Autodesk Inventor part; units mm, degrees
ref_plane "YZ Plane" through (0, 0, 0) normal (1, 0, 0) x (0, 1, 0)
ref_plane "XZ Plane" through (0, 0, 0) normal (0, 1, 0) x (-1, 0, 0)
ref_plane "XY Plane" through (0, 0, 0) normal (0, 0, 1) x (1, 0, 0)
sketch "Sketch1" plane through (0, 0, 0) normal (0, 0, 1) x (1, 0, 0)
  line L0 (-28.59, -15) -> (28.59, -15)
  line L1 (28.59, -15) -> (28.59, 15)
  line L2 (28.59, 15) -> (-28.59, 15)
  line L3 (-28.59, 15) -> (-28.59, -15)
  line L4 (-28.59, -15) -> (28.59, 15) construction
  line L5 (28.59, -15) -> (-28.59, 15) construction
  point P0 (0, 0)
  dimension "d0" = 57.18
  dimension "d1" = 30
extrude "Plate1" add sketch "Sketch1" along normal blind 1.5
sketch "Sketch2" plane through (-27.09, -15, 0) normal (-1, 0, 0) x (0, -1, 0)
  line L0 (-30, 0) -> (0, 0)
  line L1 (0, 0) -> (0, 40)
  line L2 (0, 40) -> (-30, 40)
  line L3 (-30, 40) -> (-30, 0)
edge flange "Flange1" height 40 angle 90 thickness 1.5 bend radius 0.31 thickness toward (-1, 0, 0) relief tear relief width 1.5 relief depth 0.75 corner gap 0.31 corner form 0 edges at (-28.59, 0, 1.5) (28.59, 0, 1.5) wall of the first edge with corners at (-27.09, 15, 0) (-27.09, -15, 0) (-27.09, -15, 40) (-27.09, 15, 40)
bend "Bend1"
corner "Corner1"
sketch "Sketch3" plane through (28.59, -15, 40) normal (1, 0, 0) x (0, 0, -1)
  circle A0 centre (15, 15) radius 9.96
  line L0 (0, 30) -> (38.19, 30)
  line L1 (38.19, 0) -> (0, 0)
  line L2 (38.19, 30) -> (12.9705, 24.751)
  line L3 (38.19, 0) -> (12.9705, 5.249)
  line L4 (0, 30) -> (0, 0)
  point P0 (40, 15)
  dimension "d13" = 19.92
  dimension "d14" = 0
  dimension "d15" = 25
sketch "Sketch19" plane through (0, 0, 1.5) normal (0, 0, 1) x (1, 0, 0)
  point P0 (0, 0)
sketch "Sketch21" plane through (-28.59, -15, 1.81) normal (-1, 0, 0) x (0, 0, 1)
  point P0 (-1.81, 15)
sketch "Sketch23" plane through (-28.59, -15, 1.81) normal (-1, 0, 0) x (0, 0, 1)
  point P0 (-1.81, 15)
sketch "Sketch25" plane through (0, 0, 1.5) normal (0, 0, 1) x (1, 0, 0)
  circle A0 centre (7.525, 7.5) radius 0.7835
  circle A1 centre (7.525, -12.5) radius 0.7835
  circle A2 centre (-7.525, -12.5) radius 0.7835
  circle A3 centre (-7.525, 7.5) radius 0.7835
  point P0 (0, 0)
hole "Hole12" at (7.525, 7.5, 1.5) at (7.525, -12.5, 1.5) at (-7.525, 7.5, 1.5) at (-7.525, -12.5, 1.5) direction (0, 0, -1) diameter 2.1 depth 1.5
extrude "Cut7" cut sketch "Sketch3" against normal blind 1.5 contours A0 L3 L1 L4 L0 L2
mirror "Mirror1" about plane through (0, 0, 0) normal (1, 0, 0) of "Cut7"
sketch "Sketch26" plane through (-28.59, -15, 1.81) normal (-1, 0, 0) x (0, 0, 1)
  circle A0 centre (30.19, 15) radius 0.7835
  circle A1 centre (23.19, 22) radius 0.7835
  circle A2 centre (23.19, 8) radius 0.7835
  circle A3 centre (16.19, 15) radius 0.7835
  point P0 (-1.81, 15)
hole "Hole13" at (-28.59, 0, 32) at (-28.59, 7, 25) at (-28.59, -7, 25) at (-28.59, 0, 18) direction (1, 0, 0) diameter 2.1 depth 1.5
sketch "Sketch27" plane through (-28.59, -15, 1.81) normal (-1, 0, 0) x (0, 0, 1)
  circle A0 centre (23.19, 15) radius 3
  point P0 (-1.81, 15)
hole "Hole14" at (-28.59, 0, 25) direction (1, 0, 0) diameter 7.2 depth 1.5
sketch "Sketch28" plane through (28.59, -15, 1.81) normal (1, 0, 0) x (0, 0, -1)
  circle A0 centre (-30.19, 15) radius 0.7835
  circle A1 centre (-23.19, 8) radius 0.7835
  circle A2 centre (-23.19, 22) radius 0.7835
  circle A3 centre (-16.19, 15) radius 0.7835
  point P0 (1.81, 15)
hole "Hole15" at (28.59, 0, 32) at (28.59, -7, 25) at (28.59, 0, 18) at (28.59, 7, 25) direction (-1, 0, 0) diameter 2.1 depth 1.5
sketch "Sketch29" plane through (28.59, -15, 1.81) normal (1, 0, 0) x (0, 0, -1)
  circle A0 centre (-23.19, 15) radius 1.75
  point P0 (1.81, 15)
hole "Hole16" at (28.59, 0, 25) direction (-1, 0, 0) diameter 5.2 depth 1.5
equation "\"d125\" = Thickness"
equation "\"d127\" = Thickness"
equation "\"d134\" = Thickness"
equation "\"d141\" = Thickness"
equation "\"d148\" = Thickness"
equation "\"d155\" = Thickness"
equation "\"d2\" = Thickness"
equation "\"d3\" = BendReliefWidth"
equation "\"d4\" = BendReliefDepth"
equation "\"d5\" = MinimumRemnant"
equation "\"d6\" = TransitionRadius"
equation "\"d9\" = BendRadius"
equation "\"d10\" = CornerReliefSize"
equation "\"d11\" = GapSize"
equation "\"d12\" = JacobiRadiusSize"
equation "\"BendReliefWidth\" = Thickness"
equation "\"BendReliefDepth\" = 0.5 * Thickness"
equation "\"CornerReliefSize\" = 4 * Thickness"
equation "\"MinimumRemnant\" = 2 * Thickness"
equation "\"TransitionRadius\" = BendRadius"
equation "\"JacobiRadiusSize\" = BendRadius"
equation "\"GapSize\" = Thickness"
properties part number "axis_14_bottom_frame" material "Aluminum 6061-AHC"
Source: CAD feature listing. Evaluate the final solid. Frame: model axes, mm. A direction names the side the tool comes from. Round coordinates to 2 decimals unless told otherwise and drop trailing zeros. Order: outer loops, then holes, each group sorted by start corner. A loop starts at its lowest first (then second) coordinate and runs counter-clockwise, first axis right, second up. Notation, with made-up numbers: (-15, 73.25) - (3, 73.25) arc R24 cw to (3, 83.25) - close; hole circle Ø8 at (47.25, 57). An arc over 180 degrees is marked (long way). Use a Markdown table: item, result. Add a question column.
1. Set-up query: faces 5 (the cylindrical face through (27.83, 6.68, 24)), 6 (the cylindrical face through (-27.83, -0.158, 21.403)), 7 (the flat face through (-27.09, 0, 14)). Return all of +Z, -Z, +X, -X, +Y, -Y with unobstructed straight access to the full face (end or side cutting, diameter ignored); none if empty.
2. Section query B-B (z = 18). Return the cut outline in (x, y).
3. Section query A-A (y = -12.5). Return the cut outline in (x, z) (3 decimals).
4. First-contact query: pin 1 (1.5 mm diameter, centred on x = 8, y = 9, fed in from +Z); pin 2 (1.9 mm diameter, centred on y = -7, z = 25, fed in from +X); pin 3 (10 mm diameter, centred on x = 22.5, z = 20.5, fed in from -Y). Flat tips, straight axial feed; report the tip coordinate or a pass-through.
5. Section query C-C (z = 25). Give the number of separate pieces and of enclosed holes in the cut face, then the cut area to 3 significant figures.
6. Line query: probe 1 along X at (y, z) = (-10, 19); probe 2 along Z at (x, y) = (-27.6, 0); probe 3 along Z at (x, y) = (28.2, 0). Output: solid intervals per line, ascending.
7. Mould query, pull axis Z, two halves, no side actions, for faces 1 (the cylindrical face through (-27.83, -0.32, 33)), 2 (the cylindrical face through (-28.07, -0.21, 0.54)), 3 (the flat face through (0, 0, 1.5)), 4 (the flat face through (27.09, 0, 14)). Classes: +Z half, -Z half, draft (parallel to the pull), parting line (faces both ways), or undercut.
Derived:
| question | item | result |
|---|---|---|
| 1 | face 5 | +X, -X |
| 1 | face 6 | -X |
| 1 | face 7 | +Z, +Y, -Y |
| 2 | outline | (-28.59, -11.63) - (-27.09, -11.63) - (-27.09, -1.05) - (-28.59, -1.05) - close; (-28.59, 1.05) - (-27.09, 1.05) - (-27.09, 11.63) - (-28.59, 11.63) - close; (27.09, -11.63) - (28.59, -11.63) - (28.59, -1.05) - (27.09, -1.05) - close; (27.09, 1.05) - (28.59, 1.05) - (28.59, 11.63) - (27.09, 11.63) - close |
| 3 | outline | (-28.59, 1.81) arc R1.81 ccw to (-26.78, 0) - (-8.575, 0) - (-8.575, 1.5) - (-26.78, 1.5) arc R0.31 cw to (-27.09, 1.81) - (-27.09, 13.822) - (-28.59, 13.822) - close; (-6.475, 0) - (6.475, 0) - (6.475, 1.5) - (-6.475, 1.5) - close; (8.575, 0) - (26.78, 0) arc R1.81 ccw to (28.59, 1.81) - (28.59, 13.822) - (27.09, 13.822) - (27.09, 1.81) arc R0.31 cw to (26.78, 1.5) - (8.575, 1.5) - close |
| 4 | pin 1 | z = 1.5 |
| 4 | pin 2 | through |
| 4 | pin 3 | y = -11.52 |
| 5 | separate pieces | 8 |
| 5 | enclosed holes | 0 |
| 5 | area | 29.8 mm2 |
| 6 | probe 1 | -28.59 to -27.09, 27.09 to 28.59 |
| 6 | probe 2 | 0.2 to 16.95, 19.05 to 21.4, 28.6 to 30.95, 33.05 to 34.96 |
| 6 | probe 3 | 0.69 to 16.95, 19.05 to 22.4, 27.6 to 30.95, 33.05 to 34.96 |
| 7 | face 1 | undercut |
| 7 | face 2 | -Z half |
| 7 | face 3 | +Z half |
| 7 | face 4 | draft |
